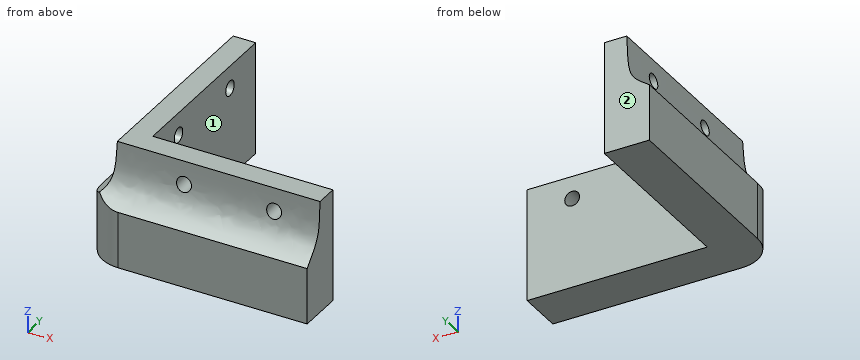
```python
from build123d import *

# Parameters (mm, degrees)
F1_DEPTH = 25
F3_DEPTH = 50.001
F5_DEPTH = 50.0010001
F7_D     = 3.3
F9_D     = 3.3


with BuildPart() as f1:
    # F0 (on Top) → F1 (new body)
    with BuildSketch(Plane.XY):
        with BuildLine():
            Line((0, 50), (0, 8))
            ThreePointArc((0, 8), (2.3431457505, 2.3431457505), (8, 0))
            Line((8, 0), (50, 0))
            Line((50, 0), (50, 10))
            Line((50, 10), (10, 10))
            Line((10, 10), (10, 50))
            Line((10, 50), (0, 50))
        make_face()
    extrude(amount=F1_DEPTH)

    # F2 (on face) → F3 (cut, through all)
    with BuildSketch(Plane.YZ.offset(50)):
        with BuildLine():
            add(Edge.make_bspline(
                [(5, 25), (4.6534377741, 17.5), (4.6950438991, 17.3452608287), (0, 12.5)],
                knots=[0, 0, 0, 0, 13.4629120178, 13.4629120178, 13.4629120178, 13.4629120178], degree=3))
            Line((5, 25), (0, 25))
            Line((0, 25), (0, 12.5))
        make_face()
    extrude(amount=-F3_DEPTH, mode=Mode.SUBTRACT)

    # F4 (on face) → F5 (cut, through all)
    with BuildSketch(Plane(origin=(0, 50, 0), x_dir=(-1, 0, 0), z_dir=(0, 1, 0))):
        with BuildLine():
            Line((0, 25), (-5, 25))
            add(Edge.make_bspline(
                [(-5, 25), (-4.6829669736, 15.6825594604), (-4.6829669736, 15.6825594604), (0, 12.5)],
                knots=[0, 0, 0, 0, 13.4629120178, 13.4629120178, 13.4629120178, 13.4629120178], degree=3))
            Line((0, 12.5), (0, 25))
        make_face()
    extrude(amount=-F5_DEPTH, mode=Mode.SUBTRACT)

    # F7 (through all)
    with Locations(Plane(origin=(0, 10, 0), x_dir=(-1, 0, 0), z_dir=(0, 1, 0))):
        with Locations((-40, 20), (-20, 20)):
            Hole(F7_D / 2)

    # F9 (through all)
    with Locations(Plane.YZ.offset(10)):
        with Locations((20, 20), (40, 20)):
            Hole(F9_D / 2)


solid = f1.part
```
Geometry: final body of the model. Coordinates: model frame, mm. Face numbers are marked on the shaded views. A direction names the side the tool comes from. Round coordinates to 2 decimals unless told otherwise and drop trailing zeros. Order: outer loops, then holes, each group sorted by start corner. A loop starts at its lowest first (then second) coordinate and runs counter-clockwise, first axis right, second up. Notation, with made-up numbers: (33.5, -4.75) -> (65.5, -4.75) arc R12 cw to (65.5, 9.25) -> close; hole circle Ø5 at (52, 78.25). An arc over 180 degrees is marked (long way). Use CSV: the item, a comma, the result in double quotes. Start each with the question number.
1) Set-up query: the marked faces 1 and 2. Return all of +Z, -Z, +X, -X, +Y, -Y with unobstructed straight access to the full face (end or side cutting, diameter ignored); none if empty.
2) Material intervals for line 1 along X through (y, z) = (5.9, 20); line 2 along Z through (x, y) = (8, 40); line 3 along Y through (x, z) = (6.65, 20), sorted ascending. Write a range as from..to.
3) First-contact query: pin 1 Ø12.5 at (x, z) = (29.5, 17.5) entering from +Y; pin 2 Ø2 at (y, z) = (22, 16) entering from -X; pin 3 Ø12.5 at (y, z) = (37, 17.5) entering from +X; pin 4 Ø1.5 at (x, y) = (27, 9.5) entering from -Z. Flat tips, straight axial feed; report the tip coordinate or a pass-through.
4) Section A-A (z = 7.75). Return the cut outline in (x, y), and give its area (3 significant figures).
5) Section B-B (z = 21). State how many separate pieces and enclosed holes the cut face has, and give its area (3 significant figures).
Returned:
1,face 1,"+Z, -Z, +X, +Y"
1,face 2,"+Z, -Z, +X, -X, +Y"
2,line 1,"x = 4.78..18.35, 21.65..38.35, 41.65..50"
2,line 2,"z = 0..18.35, 21.65..25"
2,line 3,"y = 4.67..18.35, 21.65..38.35, 41.65..50"
3,pin 1,"stops at y = 10"
3,pin 2,"stops at x = 3.23"
3,pin 3,"stops at x = 10"
3,pin 4,"stops at z = 0"
4,outline,"(0, 8) arc R8 ccw to (8, 0) -> (50, 0) -> (50, 10) -> (10, 10) -> (10, 50) -> (0, 50) -> close"
4,area,"886 mm²"
5,separate pieces,"5"
5,enclosed holes,"0"
5,area,"388 mm²"
